Source: three-view drawing plus pictorial views. Frame: mm from the lowest corner of the part. A direction names the side the tool comes from. Give positions to 0.01 mm unless a question says otherwise; leave off trailing zeros. Loops run counter-clockwise (first coordinate to the right, second up) from the corner with the lowest first, then second, coordinate; pieces in that order, holes last. Notation, with made-up numbers: M 86.25,-12 L 105.25,-12 A20 ccw 105.25,24 Z; hole C 51.5,-19 d3. An arc over 180 degrees is marked long. One line per item, written item: value. Start each with the question number.
(1) Pin query (flat end, axial travel): P1, Ø3, axis at x = 9, z = 9, coming from the +Y side; P2, Ø3, axis at y = 3.5, z = 9, coming from the -X side; P3, Ø5, axis at y = 18, z = 13, coming from the -X side. Return the tip coordinate at first contact, or that it passes through.
(2) Section C-C on z = 14.25. Output: boundary loops of the cut face in (x, y) (3 decimals).
(3) Ray query, line 1 along Y through (x, z) = (9, 17.75) (3 decimals); line 2 along Z through (x, y) = (6.35, 8.75) (3 decimals); line 3 along Y through (x, z) = (27, 12.5). Return the intervals inside material, ascending. Write a range as from..to.
(4) Section A-A on x = 4. Output: boundary loops of the cut face in (y, z) (3 decimals), plus the area to 3 significant figures.
(5) Access query for the marked faces 4, 5 and 6. Directions: +Z, -Z, +X, -X, +Y, -Y. A direction counts if a zero-diameter tool reaches every point of the face in a straight line with its end or side. Return the directions, or none.
(6) Section B-B on y = 19.9. Output: boundary loops of the cut face in (x, z) (3 decimals).
(7) Section D-D on y = 5.25. Output: boundary loops of the cut face in (x, z).
(8) Pull-direction query (Y, two-part tool) for the marked faces 1, 2 and 3; classes: released by +Y, released by -Y, zero draft, split by the parting line, or undercut.
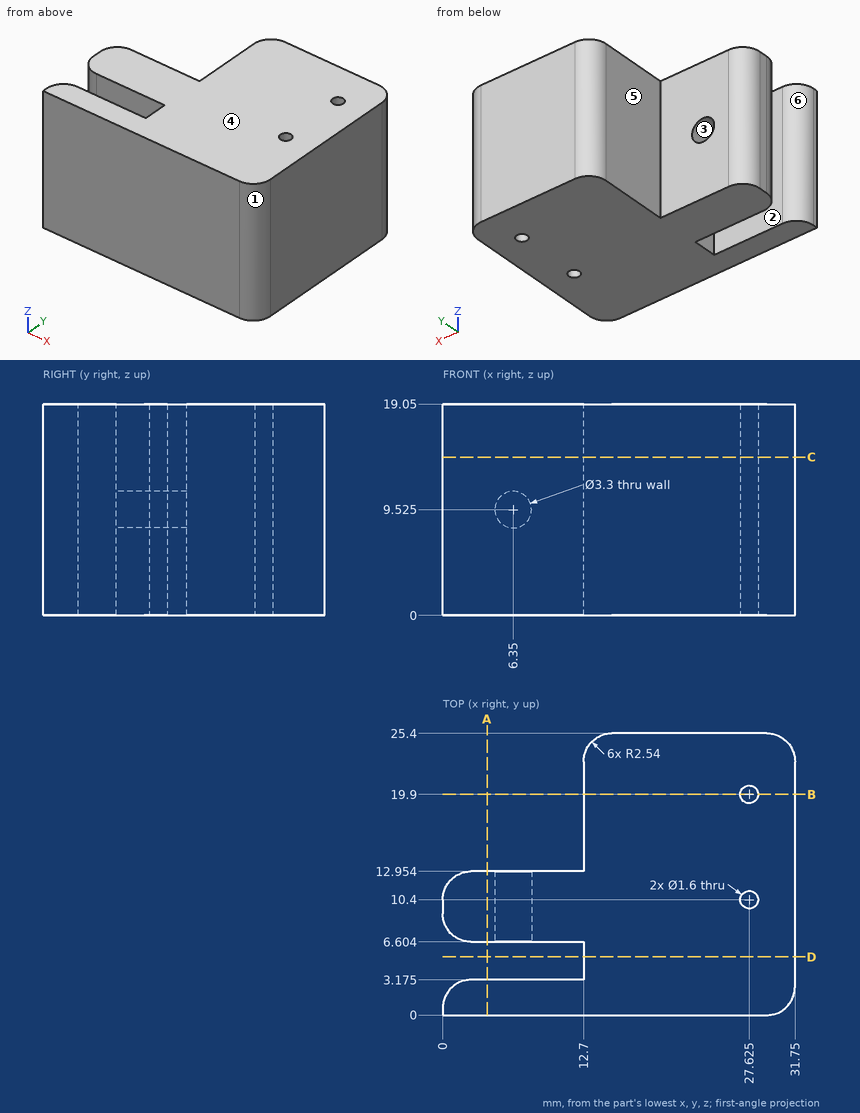
Output values:
1. P1: stops at y = 12.95
1. P2: stops at x = 0.4
1. P3: stops at x = 12.7
2. outline: M 0,0 L 29.21,0 A2.54 ccw 31.75,2.54 L 31.75,22.86 A2.54 ccw 29.21,25.4 L 15.24,25.4 A2.54 ccw 12.7,22.86 L 12.7,12.954 L 2.54,12.954 A2.54 ccw 0,10.414 L 0,9.144 A2.54 ccw 2.54,6.604 L 12.7,6.604 L 12.7,3.175 L 2.54,3.175 A2.54 ccw 0,0.635 Z; hole C 27.625,10.4 d1.6; hole C 27.625,19.9 d1.6
3. line 1: y = 0..3.175, 6.604..12.954
3. line 2: z = 0..7.875, 11.175..19.05
3. line 3: y = 0..9.9, 10.9..19.4, 20.4..25.4
4. outline: M 0,0 L 3.175,0 L 3.175,19.05 L 0,19.05 Z; M 6.604,0 L 12.954,0 L 12.954,19.05 L 6.604,19.05 Z
4. area: 181 mm²
5. face 4: +Z, +X, -X, +Y, -Y
5. face 5: +Z, -Z, -X, +Y
5. face 6: +Z, -Z, -X
6. outline: M 12.7,0 L 26.825,0 L 26.825,19.05 L 12.7,19.05 Z; M 28.425,0 L 31.75,0 L 31.75,19.05 L 28.425,19.05 Z
7. outline: M 12.7,0 L 31.75,0 L 31.75,19.05 L 12.7,19.05 Z
8. face 1: released by -Y
8. face 2: undercut
8. face 3: zero draft
